For this review, use the dimensioned drawing (mm, ordinates from the lowest corner) and the shaded views. Give positions to 0.01 mm unless a question says otherwise; leave off trailing zeros. Loops run counter-clockwise (first coordinate to the right, second up) from the corner with the lowest first, then second, coordinate; pieces in that order, holes last. Notation, with made-up numbers: (-37.75, 34.25) -> (-29.75, 34.25) arc R14 ccw to (-29.75, 46.25) -> close; hole circle Ø6 at (13.25, 74.5). An arc over 180 degrees is marked (long way). Write each question's results on one line, items separated by ' | '. Start each with the question number.
Q1. We need section C-C (z = 1.85). Give the number of separate pieces and of enclosed holes in the cut face, plus the area to 3 significant figures.
Q2. We need section A-A (x = 23). Write out the cut boundary in (y, z), plus the area to 3 significant figures.
Q3. We need section B-B (y = 41.5). Write out the cut boundary in (x, z).
Q4. Wall thickness on L1, parallel to Y at x = 14, z = 2.25; L2, parallel to Y at x = 36, z = 1.1; L3, parallel to X at y = 29.5, z = 1.95: over which ranges is each line inside the solid? List them lowest first. Write a range as [from, to].
Q5. Insertion check: pin 1 Ø1.6 at (x, y) = (14, 4) entering from -Z. The pin has a flat end and moves straight along its axis. Give the tip position at first contact, or say it passes through.
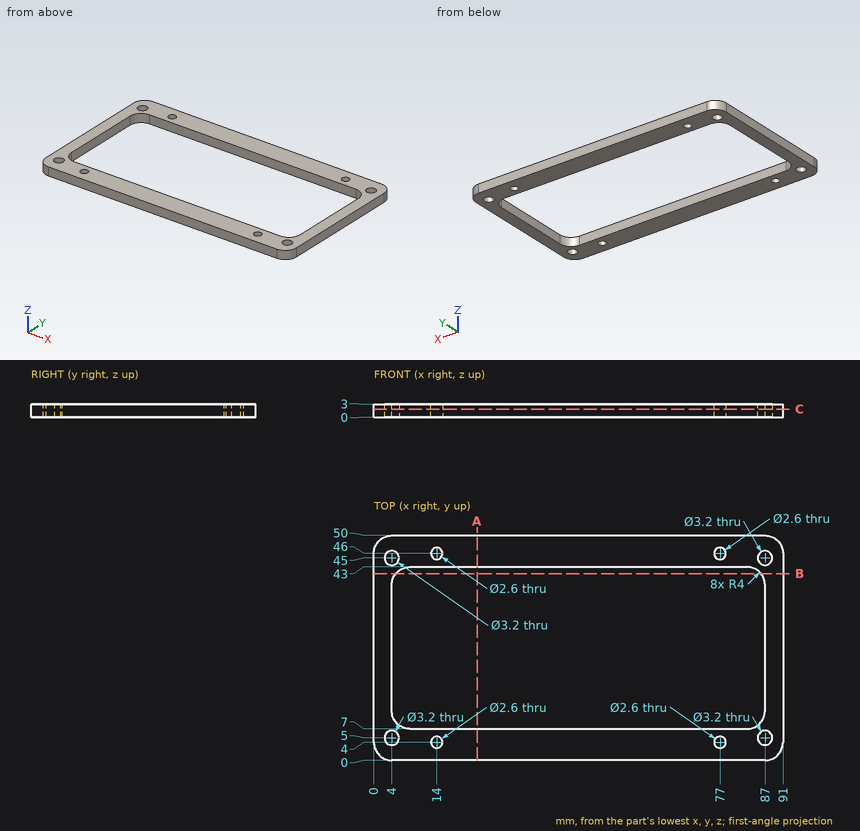
Output:
1) separate pieces: 1 | enclosed holes: 9 | area: 1,510 mm2
2) outline: (0, 0) -> (7, 0) -> (7, 3) -> (0, 3) -> close; (43, 0) -> (50, 0) -> (50, 3) -> (43, 3) -> close | area: 42.0 mm2
3) outline: (0, 0) -> (4.88, 0) -> (4.88, 3) -> (0, 3) -> close; (86.12, 0) -> (91, 0) -> (91, 3) -> (86.12, 3) -> close
4) L1: [0, 2.7], [5.3, 7], [43, 44.7], [47.3, 50] | L2: [0, 7], [43, 50] | L3: [0, 4], [87, 91]
5) pin 1: through
